```python
from build123d import *

# Parameters (mm, degrees)
F0_W     = 5.842
F0_H     = 12.7
F0_R     = 3.175
F2_DEPTH = 6.35
F3_R     = 1.524
F4_DEPTH = 6.35
F5_DEPTH = 7.62


with BuildPart() as f1:
    # F0 (on Front) → F1 (revolve)
    with BuildSketch(Plane.XZ):
        Polygon((5.842, 12.7), (5.842, 0), (66.294, 0), (66.294, 12.7), (56.134, 12.7), (56.134, 10.16), (10.16, 10.16), (10.16, 12.7), align=None)
        with Locations((2.921, 6.35)):
            Rectangle(F0_W, F0_H)
    revolve(axis=Axis((33.147, 0, 0), (-1, 0, 0)))

    # F0 (on Front) → F2 (join)
    with BuildSketch(Plane.XZ):
        with BuildLine():
            Line((-0.9398, 0), (0, 0))
            Line((0, 0), (0, 12.7))
            Line((0, 12.7), (5.842, 12.7))
            Line((5.842, 12.7), (5.842, 15.24))
            Line((5.842, 15.24), (-0.508, 15.24))
            Line((-0.508, 15.24), (-10.8806298187, 3.8475430269))
            ThreePointArc((-10.8806298187, 3.8475430269), (-4.5919612295, 5.3297205562), (-0.9398, 0))
        make_face()
        with BuildLine():
            Line((5.842, 0), (0, 0))
            Line((0, 0), (-0.9398, 0))
            ThreePointArc((-0.9398, 0), (-3.1957909266, -4.5493385486), (-8.1826630726, -5.5069827884))
            Line((-8.1826630726, -5.5069827884), (5.842, -9.398))
            Line((5.842, -9.398), (5.842, 0))
        make_face()
        with Locations((2.921, 6.35)):
            Rectangle(F0_W, F0_H)
        with BuildLine():
            ThreePointArc((-8.1826630726, -5.5069827884), (-3.1957909266, -4.5493385486), (-0.9398, 0))
            ThreePointArc((-0.9398, 0), (-4.5919612295, 5.3297205562), (-10.8806298187, 3.8475430269))
            ThreePointArc((-10.8806298187, 3.8475430269), (-12.1459778134, -1.5837270034), (-8.1826630726, -5.5069827884))
        make_face()
        with Locations((-6.6548, 0)):
            Circle(F0_R, mode=Mode.SUBTRACT)
    extrude(amount=F2_DEPTH)

    # F3 (on face) → F4 (join)
    with BuildSketch(Plane.YZ.offset(66.294)):
        with BuildLine():
            ThreePointArc((-5.08, 11.6397422652), (0, 12.7), (5.08, 11.6397422652))
            Line((5.08, 11.6397422652), (5.08, 15.24))
            Line((5.08, 15.24), (-5.08, 15.24))
            Line((-5.08, 15.24), (-5.08, 11.6397422652))
        make_face()
        with BuildLine():
            ThreePointArc((-5.08, 0), (0, 5.08), (5.08, 0))
            Line((5.08, 0), (5.08, 11.6397422652))
            ThreePointArc((5.08, 11.6397422652), (0, 12.7), (-5.08, 11.6397422652))
            Line((-5.08, 11.6397422652), (-5.08, 0))
        make_face()
        with BuildLine():
            ThreePointArc((-5.08, 0), (0, -5.08), (5.08, 0))
            ThreePointArc((5.08, 0), (0, 5.08), (-5.08, 0))
        make_face()
        Circle(F3_R, mode=Mode.SUBTRACT)
    extrude(amount=F4_DEPTH)

    # F5 (add): a face of the model
    f5_faces = [f1.faces().sort_by_distance(p)[0] for p in [
        (72.644, 0, 5.8085929676),
    ]]
    extrude(f5_faces, amount=-F5_DEPTH)


solid = f1.part
```
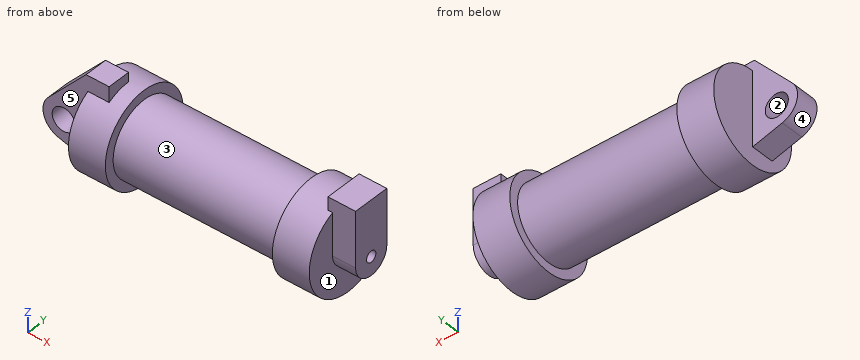
Source: CAD feature listing. Evaluate the final solid. Frame: model axes, mm. Face numbers are marked on the shaded views. A direction names the side the tool comes from. Give positions to 0.01 mm unless a question says otherwise; leave off trailing zeros. Loops run counter-clockwise (first coordinate to the right, second up) from the corner with the lowest first, then second, coordinate; pieces in that order, holes last. Notation, with made-up numbers: (11, 44.25) -> (56, 44.25) arc R20 cw to (56, 74.25) -> close; hole circle Ø10 at (36.25, 78). An arc over 180 degrees is marked (long way). Use a Markdown table: item, result. Add a question column.
(1) Access query for the marked faces 1 and 2. Directions: +Z, -Z, +X, -X, +Y, -Y. A direction counts if a zero-diameter tool reaches every point of the face in a straight line with its end or side. Return the directions, or none.
(2) Pull-direction query (X, two-part tool) for the marked faces 3, 4 and 5; classes: +X half, -X half, draft (parallel to the pull), parting line (faces both ways), or undercut.
(3) Section query C-C (x = 22.5). Output: boundary loops of the cut face in (y, z).
(4) Section query B-B (y = 11.25). Output: boundary loops of the cut face in (x, z), then the cut area to 3 significant figures.
(5) Section query D-D (z = 9). Output: boundary loops of the cut face in (x, y), then the cut area to 3 significant figures.
(6) Section query A-A (y = -4). Output: boundary loops of the cut face in (x, z) (3 decimals).
(7) Ray query, line 1 (Y direction, x = 68, z = 4); line 2 (Z direction, x = 68, y = 0); line 3 (X direction, y = 6.25, z = -0.25). Return the intervals inside material, ascending.
(8) First-contact query: pin 1 Ø5.5 at (x, z) = (-6.65, 0) entering from -Y; pin 2 Ø6 at (x, z) = (67.5, 11.5) entering from +Y; pin 3 Ø4 at (y, z) = (-7.5, -6.5) entering from +X; pin 4 Ø4 at (y, z) = (4.5, -8) entering from -X. Flat tips, straight axial feed; report the tip coordinate or a pass-through.
Checked values:
| question | item | result |
|---|---|---|
| 1 | face 1 | -Z, +X |
| 1 | face 2 | +Y, -Y |
| 2 | face 3 | undercut |
| 2 | face 4 | -X half |
| 2 | face 5 | draft |
| 3 | outline | circle Ø20.32 at (0, 0) |
| 4 | outline | (0, -5.89) -> (10.16, -5.89) -> (10.16, 5.89) -> (0, 5.89) -> close; (56.13, -5.89) -> (66.29, -5.89) -> (66.29, 5.89) -> (56.13, 5.89) -> close |
| 4 | area | 239 mm^2 |
| 5 | outline | (-6.19, -6.35) -> (0, -6.35) -> (0, -8.96) -> (10.16, -8.96) -> (10.16, -4.71) -> (56.13, -4.71) -> (56.13, -8.96) -> (66.29, -8.96) -> (66.29, -5.08) -> (72.64, -5.08) -> (72.64, 5.08) -> (66.29, 5.08) -> (66.29, 8.96) -> (56.13, 8.96) -> (56.13, 4.71) -> (10.16, 4.71) -> (10.16, 8.96) -> (0, 8.96) -> (0, 0) -> (-6.19, 0) -> close |
| 5 | area | 901 mm^2 |
| 6 | outline | (-10.881, 3.848) arc R5.715 ccw to (-8.183, -5.507) -> (0, -7.777) -> (0, -12.054) -> (10.16, -12.054) -> (10.16, -9.339) -> (56.134, -9.339) -> (56.134, -12.054) -> (66.294, -12.054) -> (66.294, -3.132) -> (72.644, -3.132) -> (72.644, 15.24) -> (65.024, 15.24) -> (65.024, 12.054) -> (56.134, 12.054) -> (56.134, 9.339) -> (10.16, 9.339) -> (10.16, 12.054) -> (5.842, 12.054) -> (5.842, 15.24) -> (-0.508, 15.24) -> close; hole circle Ø6.35 at (-6.655, 0) |
| 7 | line 1 | -5.08 to 5.08 |
| 7 | line 2 | -5.08 to -1.52, 1.52 to 15.24 |
| 7 | line 3 | 0 to 66.29 |
| 8 | pin 1 | through |
| 8 | pin 2 | y = 9.2 |
| 8 | pin 3 | x = 66.29 |
| 8 | pin 4 | x = 0 |
